Geometry: final body of the model. Coordinates: model frame, mm. A direction names the side the tool comes from. Give positions to 0.01 mm unless a question says otherwise; leave off trailing zeros. Write each loop counter-clockwise with the first axis right and the second up, starting at its lowest first coordinate (ties: lowest second). Pieces come first, ordered by that corner, then holes. Notation, with made-up numbers: (19.25, 73.25) -> (64.25, 73.25) arc R4 cw to (64.25, 80.25) -> close; hole circle Ø1 at (66, 15). An arc over 180 degrees is marked (long way). Answer as a JSON object with one key per item and string values.
from build123d import *

# Parameters (mm, degrees)
CROQUIS1_W              = 22
CROQUIS1_H              = 23
SALIENTE_EXTRUIR1_DEPTH = 12
CROQUIS2_W              = 12
CROQUIS2_H              = 2
SALIENTE_EXTRUIR2_DEPTH = 5
CORTAR_EXTRUIR2_DEPTH   = 2
CROQUIS13_W             = 12
CROQUIS13_H             = 2
SALIENTE_EXTRUIR3_DEPTH = 4
CORTAR_EXTRUIR3_DEPTH   = 2
SALIENTE_EXTRUIR4_DEPTH = 4
CROQUIS16_R             = 2.5
SALIENTE_EXTRUIR5_DEPTH = 6
CROQUIS21_R             = 0.75
CORTAR_EXTRUIR6_DEPTH   = 2


with BuildPart() as part:
    # Croquis1 → Saliente-Extruir1 (new body)
    with BuildSketch(Plane.XY):
        with Locations((-25.140327955, -0.424857882)):
            Rectangle(CROQUIS1_W, CROQUIS1_H)
    extrude(amount=SALIENTE_EXTRUIR1_DEPTH)

    # Croquis2 → Saliente-Extruir2 (add)
    with BuildSketch(Plane(origin=(-14.140327955, 0, 0), x_dir=(0, 0, -1), z_dir=(1, 0, 0))):
        with Locations((-6, 6.075142118)):
            Rectangle(CROQUIS2_W, CROQUIS2_H)
    saliente_extruir2 = extrude(amount=SALIENTE_EXTRUIR2_DEPTH)

    # Croquis3 → Cortar-Extruir2 (cut)
    with BuildSketch(Plane(origin=(0, 7.075142118, 0), x_dir=(1, 0, 0), z_dir=(0, 1, 0))):
        with BuildLine():
            Line((-10.140327955, -5.5), (-10.726114393, -5.5))
            ThreePointArc((-10.726114393, -5.5), (-13.640327955, -6), (-10.726114393, -6.5))
            Line((-10.726114393, -6.5), (-10.140327955, -6.5))
            Line((-10.140327955, -6.5), (-10.140327955, -12))
            Line((-10.140327955, -12), (-9.140327955, -12))
            Line((-9.140327955, -12), (-9.140327955, 0))
            Line((-9.140327955, 0), (-10.140327955, 0))
            Line((-10.140327955, 0), (-10.140327955, -5.5))
        make_face()
    cortar_extruir2 = extrude(amount=-CORTAR_EXTRUIR2_DEPTH, mode=Mode.SUBTRACT)

    # Simetría1: Saliente-Extruir2, Cortar-Extruir2 across plane
    add(saliente_extruir2.mirror(Plane(origin=(-9.140327955, 7.075142118, 12), x_dir=(0, 0, 1), z_dir=(0, -1, 0))))
    add(cortar_extruir2.mirror(Plane(origin=(-9.140327955, 7.075142118, 12), x_dir=(0, 0, 1), z_dir=(0, -1, 0))), mode=Mode.SUBTRACT)

    # Croquis13 → Saliente-Extruir3 (add)
    with BuildSketch(Plane.ZY.offset(36.140327955)):
        with Locations((6, 6.075142118)):
            Rectangle(CROQUIS13_W, CROQUIS13_H)
    extrude(amount=SALIENTE_EXTRUIR3_DEPTH)

    # Croquis14 → Cortar-Extruir3 (cut)
    with BuildSketch(Plane(origin=(0, 7.075142118, 0), x_dir=(1, 0, 0), z_dir=(0, 1, 0))):
        with BuildLine():
            Line((-40.140327955, -6.5), (-40.140327955, -5.5))
            Line((-40.140327955, -5.5), (-39.554541518, -5.5))
            ThreePointArc((-39.554541518, -5.5), (-36.640327955, -6), (-39.554541518, -6.5))
            Line((-39.554541518, -6.5), (-40.140327955, -6.5))
        make_face()
    extrude(amount=-CORTAR_EXTRUIR3_DEPTH, mode=Mode.SUBTRACT)

    # Croquis15 → Saliente-Extruir4 (add)
    with BuildSketch(Plane(origin=(0, 11.075142118, 0), x_dir=(1, 0, 0), z_dir=(0, 1, 0))):
        with BuildLine():
            ThreePointArc((-25.594684013, -3.5), (-14.140327955, -6), (-25.594684013, -8.5))
            Line((-25.594684013, -8.5), (-26.140327955, -8.5))
            ThreePointArc((-26.140327955, -8.5), (-28.640327955, -6), (-26.140327955, -3.5))
            Line((-26.140327955, -3.5), (-25.594684013, -3.5))
        make_face()
    extrude(amount=SALIENTE_EXTRUIR4_DEPTH)

    # Croquis16 → Saliente-Extruir5 (add)
    with BuildSketch(Plane(origin=(0, 11.075142118, 0), x_dir=(1, 0, 0), z_dir=(0, 1, 0))):
        with Locations(Location((-20.140327955, -6, 0), (0, 0, 270))):
            Circle(CROQUIS16_R)
    extrude(amount=SALIENTE_EXTRUIR5_DEPTH)

    # Croquis21 → Cortar-Extruir6 (cut)
    with BuildSketch(Plane(origin=(0, 17.075142118, 0), x_dir=(1, 0, 0), z_dir=(0, 1, 0))):
        with Locations(Location((-20.140327955, -6, 0), (0, 0, 270))):
            Circle(CROQUIS21_R)
    extrude(amount=-CORTAR_EXTRUIR6_DEPTH, mode=Mode.SUBTRACT)


solid = part.part
Q1. Set-up query: faces 1 (the flat face through (-16, 11.075, 1)), 2 (the flat face through (-36.14, -4, 6)), 3 (the flat face through (-37.2, 7.075, 4.6)), 4 (the cylindrical face through (-14.145, 13.047, 5.772)), 5 (the flat face through (-13.1, 9.075, 7.4)). Return all of +Z, -Z, +X, -X, +Y, -Y with unobstructed straight access to the full face (end or side cutting, diameter ignored); none if empty.
Values:
{"face 1": "-Z, +X, +Y", "face 2": "+Z, -Z, -X, -Y", "face 3": "+Z, -Z, -X, +Y", "face 4": "+Y", "face 5": "+Z, -Z, +X, +Y"}
Q2. Mould query, pull axis X, two halves, no side actions, for faces 6 (the cylindrical face through (-36.64, 6.09, 5.94)), 7 (the flat face through (-21, 17.075, 5)), 8 (the flat face through (-36.14, 9, 6)). Classes: pulls with the +X half, pulls with the -X half, needs draft (parallel to the pull), parting line crosses it, or undercut.
Values:
{"face 6": "undercut", "face 7": "needs draft", "face 8": "pulls with the -X half"}
Q3. Material intervals for L1, parallel to X at y = 16.6, z = 6; L2, parallel to Y at x = -32.5, z = 2.5; L3, parallel to X at y = 6.2, z = 6, sorted ascending. Write a range as from..to.
Values:
{"L1": "-22.64..-20.89, -19.39..-17.64", "L2": "-11.92..11.08", "L3": "-36.64..-13.64"}
Q4. First-contact query: P1, Ø1.5, axis at x = -25.5, z = 8.5, coming from the +Y side; P2, Ø1.2, axis at y = 8.5, z = 6.5, coming from the -X side; P3, Ø1.2, axis at x = -37.5, z = 8, coming from the -Y side. Flat tips, straight axial feed; report the tip coordinate or a pass-through.
Values:
{"P1": "y = 15.08", "P2": "x = -36.14", "P3": "y = 5.08"}
Q5. Cut plane A-A (x = -13). Return the cut outline in (y, z).
Values:
{"outline": "(5.08, 0) -> (9.08, 0) -> (9.08, 4.77) -> (5.08, 4.77) -> close; (5.08, 7.23) -> (9.08, 7.23) -> (9.08, 12) -> (5.08, 12) -> close"}
Q6. Cut plane B-B (y = 5.5). Return the cut outline in (x, z), and give its area (3 significant figures).
Values:
{"outline": "(-40.14, 0) -> (-10.14, 0) -> (-10.14, 5.5) -> (-10.73, 5.5) arc R1.5 cw (long way) to (-10.73, 6.5) -> (-10.14, 6.5) -> (-10.14, 12) -> (-40.14, 12) -> (-40.14, 6.5) -> (-39.55, 6.5) arc R1.5 cw (long way) to (-39.55, 5.5) -> (-40.14, 5.5) -> close", "area": "345 mm²"}
Q7. Cut plane C-C (x = -33). Return the cut outline in (y, z).
Values:
{"outline": "(-11.92, 0) -> (11.08, 0) -> (11.08, 12) -> (-11.92, 12) -> close"}
Q8. Cut plane D-D (z = 8). Return the cut outline in (x, y), and give its area (3 significant figures).
Values:
{"outline": "(-40.14, 5.08) -> (-36.14, 5.08) -> (-36.14, -11.92) -> (-14.14, -11.92) -> (-14.14, 5.08) -> (-10.14, 5.08) -> (-10.14, 9.08) -> (-14.14, 9.08) -> (-14.14, 11.08) -> (-14.48, 11.08) -> (-14.48, 15.08) -> (-18.64, 15.08) -> (-18.64, 17.08) -> (-21.64, 17.08) -> (-21.64, 15.08) -> (-27.64, 15.08) -> (-27.64, 11.08) -> (-36.14, 11.08) -> (-36.14, 7.08) -> (-40.14, 7.08) -> close", "area": "589 mm²"}
